Answer from the drawing. Dimensions are ordinates in mm from the lowest x, y and z of the part. A direction names the side the tool comes from. Round coordinates to 2 decimals unless told otherwise and drop trailing zeros. Write each loop counter-clockwise with the first axis right and the second up, starting at its lowest first coordinate (ties: lowest second). Pieces come first, ordered by that corner, then holes. Notation, with made-up numbers: (-4.5, -25) - (51.5, -25) arc R24 cw to (51.5, 8) - close; hole circle Ø9 at (67, 67). An arc over 180 degrees is marked (long way). Use a Markdown table: item, result. Add a question column.
1) A cutting plane is placed at D-D (y = 19). Give the vertices of the cut face in (x, z), then the cut area to 3 significant figures.
2) Each of these flat-tipped pins is pushed along its axis until it touches: P1, Ø8, axis at x = 40, y = 27, coming from the +Z side; P2, Ø5.5, axis at x = 54.5, y = 50, coming from the +Z side. Where does it stop, or does it pass through?
3) A cutting plane is placed at C-C (y = 50.5). Give the vertices of the cut face in (x, z), then the cut area to 3 significant figures.
4) A cutting plane is placed at B-B (x = 21). Give the vertices of the cut face in (y, z).
5) Find the intervals of material crossed by probe 1 along X at (y, z) = (55.5, 66.5); probe 2 along Z at (x, y) = (63.5, 53.5); probe 3 along Z at (x, y) = (30.5, 30), in increasing order. Write a range as from..to.
6) A tool of negligible diameter and unlimited length cuts with its end or side. For the marked faces 4, 5 and 6, from which of +Z, -Z, +X, -X, +Y, -Y can it reach the whole face along a straight path? Write none if from no direction.
7) Determine the mould class of the marked faces 1, 2 and 3 for opening direction X: +X half, -X half, draft (parallel to the pull), parting line (faces both ways), or undercut.
8) A cutting plane is placed at A-A (z = 63.5). Give the vertices of the cut face in (x, y).
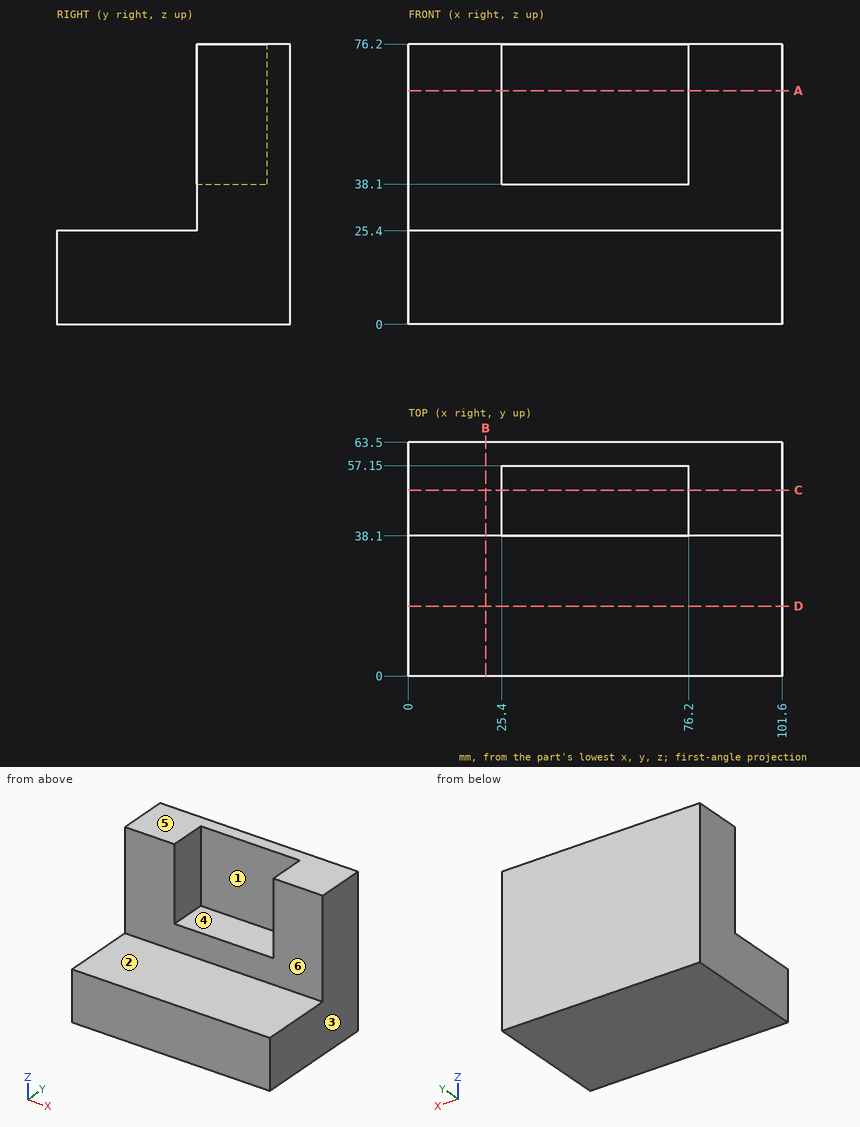
Entries:
| question | item | result |
|---|---|---|
| 1 | outline | (0, 0) - (101.6, 0) - (101.6, 25.4) - (0, 25.4) - close |
| 1 | area | 2,580 mm² |
| 2 | P1 | stops at z = 25.4 |
| 2 | P2 | stops at z = 38.1 |
| 3 | outline | (0, 0) - (101.6, 0) - (101.6, 76.2) - (76.2, 76.2) - (76.2, 38.1) - (25.4, 38.1) - (25.4, 76.2) - (0, 76.2) - close |
| 3 | area | 5,810 mm² |
| 4 | outline | (0, 0) - (63.5, 0) - (63.5, 76.2) - (38.1, 76.2) - (38.1, 25.4) - (0, 25.4) - close |
| 5 | probe 1 | x = 0..25.4, 76.2..101.6 |
| 5 | probe 2 | z = 0..38.1 |
| 5 | probe 3 | z = 0..25.4 |
| 6 | face 4 | +Z, -Y |
| 6 | face 5 | +Z, +X, -X, +Y, -Y |
| 6 | face 6 | +Z, +X, -X, -Y |
| 7 | face 1 | undercut |
| 7 | face 2 | draft |
| 7 | face 3 | +X half |
| 8 | outline | (0, 38.1) - (25.4, 38.1) - (25.4, 57.15) - (76.2, 57.15) - (76.2, 38.1) - (101.6, 38.1) - (101.6, 63.5) - (0, 63.5) - close |
